from build123d import *

# Parameters (mm, degrees)
ESQUISSE1_W             = 48
ESQUISSE1_H             = 45
BOSS_EXTRU_1_DEPTH      = 7.5
ESQUISSE2_R             = 1.75
ENL_V_MAT_EXTRU_1_DEPTH = 7
ESQUISSE3_R             = 1.75
ENL_V_MAT_EXTRU_2_DEPTH = 7
ESQUISSE5_R             = 5.5
ENL_V_MAT_EXTRU_3_DEPTH = 5
ESQUISSE4_R             = 8
ENL_V_MAT_EXTRU_4_DEPTH = 2.5


with BuildPart() as part:
    # Esquisse1 → Boss.-Extru.1 (new body)
    with BuildSketch(Plane.XY):
        Rectangle(ESQUISSE1_W, ESQUISSE1_H)
    extrude(amount=BOSS_EXTRU_1_DEPTH)

    # Esquisse2 → Enlèv. mat.-Extru.1 (cut)
    with BuildSketch(Plane.XZ.offset(22.5)):
        with Locations((-20.75, 3.75)):
            Circle(ESQUISSE2_R)
        with Locations((20.75, 3.75)):
            Circle(ESQUISSE2_R)
    extrude(amount=-ENL_V_MAT_EXTRU_1_DEPTH, mode=Mode.SUBTRACT)

    # Esquisse3 → Enlèv. mat.-Extru.2 (cut)
    with BuildSketch(Plane(origin=(0, 22.5, 0), x_dir=(1, 0, 0), z_dir=(0, 1, 0))):
        with Locations((-20.75, -3.75)):
            Circle(ESQUISSE3_R)
        with Locations((20.75, -3.75)):
            Circle(ESQUISSE3_R)
    extrude(amount=-ENL_V_MAT_EXTRU_2_DEPTH, mode=Mode.SUBTRACT)

    # Esquisse5 → Enlèv. mat.-Extru.3 (cut)
    with BuildSketch(Plane.XY.offset(7.5)):
        with Locations((0, -4.5)):
            Circle(ESQUISSE5_R)
    extrude(amount=-ENL_V_MAT_EXTRU_3_DEPTH, mode=Mode.SUBTRACT)

    # Esquisse4 → Enlèv. mat.-Extru.4 (cut)
    with BuildSketch(Plane(origin=(0, 0, 0), x_dir=(-1, 0, 0), z_dir=(0, 0, -1))):
        with Locations((0, -4.5)):
            Circle(ESQUISSE4_R)
    extrude(amount=-ENL_V_MAT_EXTRU_4_DEPTH, mode=Mode.SUBTRACT)


solid = part.part
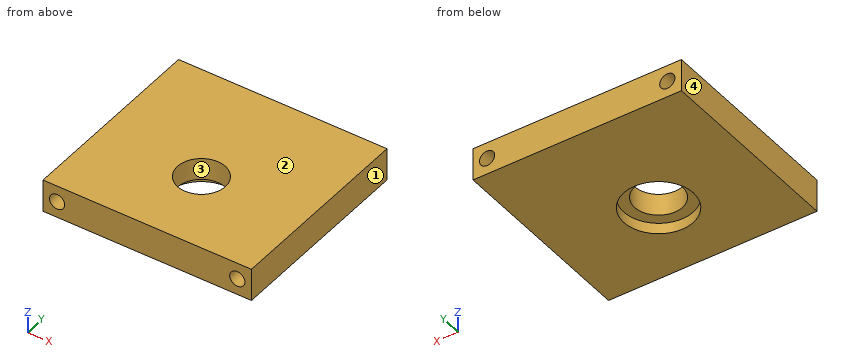
Geometry: final body of the model. Coordinates: model frame, mm. Face numbers are marked on the shaded views. Coordinates: 2 decimals unless noted, no trailing zeros. Order: outer loops, then holes, each group sorted by start corner. A loop starts at its lowest first (then second) coordinate and runs counter-clockwise, first axis right, second up.
(1) Section query C-C (z = 3.75). Return the cut outline in (x, y).
(2) Section query D-D (x = 20.75). Return the cut outline in (y, z).
(3) First-contact query: pin 1 (1 mm diameter, centred on x = 21, z = 4, fed in from +Y); pin 2 (6.5 mm diameter, centred on x = 0, y = -4.5, fed in from -Z). Flat tips, straight axial feed; report the tip coordinate or a pass-through.
(4) Material intervals for probe 1 along X at (y, z) = (19, 3.75); probe 2 along Y at (x, z) = (0, 1.3); probe 3 along Z at (x, y) = (-20.75, 18), sorted ascending.
(5) Section query A-A (x = 0). Return the cut outline in (y, z).
(6) Draft query along X for the marked faces 1, 2, 3 and 4. Return one class per face: pulls with the +X half, pulls with the -X half, needs draft (parallel to the pull), parting line crosses it, or undercut.
(7) Section query B-B (y = -4.5). Return the cut outline in (x, z), plus the area to 3 significant figures.
Solution:
1. outline: (-24, -22.5) - (-22.5, -22.5) - (-22.5, -15.5) - (-19, -15.5) - (-19, -22.5) - (19, -22.5) - (19, -15.5) - (22.5, -15.5) - (22.5, -22.5) - (24, -22.5) - (24, 22.5) - (22.5, 22.5) - (22.5, 15.5) - (19, 15.5) - (19, 22.5) - (-19, 22.5) - (-19, 15.5) - (-22.5, 15.5) - (-22.5, 22.5) - (-24, 22.5) - close; hole circle Ø11 at (0, -4.5)
2. outline: (-22.5, 0) - (22.5, 0) - (22.5, 2) - (15.5, 2) - (15.5, 5.5) - (22.5, 5.5) - (22.5, 7.5) - (-22.5, 7.5) - (-22.5, 5.5) - (-15.5, 5.5) - (-15.5, 2) - (-22.5, 2) - close
3. pin 1: stops at y = 15.5
3. pin 2: passes through
4. probe 1: x = -24 to -22.5, -19 to 19, 22.5 to 24
4. probe 2: y = -22.5 to -12.5, 3.5 to 22.5
4. probe 3: z = 0 to 2, 5.5 to 7.5
5. outline: (-22.5, 0) - (-12.5, 0) - (-12.5, 2.5) - (-10, 2.5) - (-10, 7.5) - (-22.5, 7.5) - close; (1, 2.5) - (3.5, 2.5) - (3.5, 0) - (22.5, 0) - (22.5, 7.5) - (1, 7.5) - close
6. face 1: pulls with the +X half
6. face 2: needs draft
6. face 3: undercut
6. face 4: pulls with the -X half
7. outline: (-24, 0) - (-8, 0) - (-8, 2.5) - (-5.5, 2.5) - (-5.5, 7.5) - (-24, 7.5) - close; (5.5, 2.5) - (8, 2.5) - (8, 0) - (24, 0) - (24, 7.5) - (5.5, 7.5) - close
7. area: 265 mm2
